Read the model definition and answer for the solid it produces. Units are mm, in the model's axes. A direction names the side the tool comes from. Coordinates: 2 decimals unless noted, no trailing zeros. Write each loop counter-clockwise with the first axis right and the second up, starting at its lowest first coordinate (ties: lowest second). Pieces come first, ordered by that corner, then holes. Notation, with made-up numbers: (79, 78.5) -> (100, 78.5) arc R14 ccw to (100, 85.5) -> close; hole circle Ø4 at (-7, 71). An arc over 180 degrees is marked (long way). Answer as a JSON object with one key per item and string values. Group by question number.
(1) Find section A-A (z = -38.5). Give the vertices of the cut face in (x, y), then the cut area to 3 significant figures.
(2) Find section B-B (x = 160.5). Give the vertices of the cut face in (y, z).
(3) Find section C-C (y = 30.5). Give the vertices of the cut face in (x, z), then the cut area to 3 significant figures.
(4) Which of the six approach directions +Z, -Z, +X, -X, +Y, -Y give full straight-line access (tool end or side, diameter ignored) to faces 5 (the face through (148, 44.45, -50)), 6 (the face through (246.77, 3.13, -29.3)), 7 (the face through (260.63, 27.88, -98.47)), 8 (the face through (254.514, 26.016, -3.131))?
(5) For a pull along Z with two mould halves and no side action, classify faces 1 (the face through (148, 0, -52)), 2 (the face through (246.619, 3.131, -72.715)), 3 (the face through (148, 26, -101.6)), 4 (the face through (148, 25, 0)) as +Z half, -Z half, draft (parallel to the pull), parting line (faces both ways), or undercut.
(6) Straight lines are drawn through the part: L1, parallel to Z at x = 242, y = 2; L2, parallel to Y at x = 287, z = -4; L3, parallel to X at y = 47.25, z = -30.8. For each, find the intervals that lie inside material, in ascending order.
(7) Flat-ended cylindrical pins translate along their axes: P1, Ø9, axis at x = 242, z = -70.8, coming from the -Y side; P2, Ø3.5, axis at x = 255.065, y = 38.835, coming from the +Z side. Find the tip coordinate at first contact, or state that the pin passes through.
Autodesk Inventor part; units mm, degrees
ref_plane "YZ Plane" through (0, 0, 0) normal (1, 0, 0) x (0, 1, 0)
ref_plane "XZ Plane" through (0, 0, 0) normal (0, 1, 0) x (-1, 0, 0)
ref_plane "XY Plane" through (0, 0, 0) normal (0, 0, 1) x (1, 0, 0)
sketch "Sketch1" plane through (0, 0, 0) normal (1, 0, 0) x (0, 1, 0)
  line L0 (0, 0) -> (50.8, 0)
  line L1 (50.8, 0) -> (50.8, -101.6)
  line L2 (50.8, -101.6) -> (0, -101.6)
  line L3 (0, -101.6) -> (0, 0)
  dimension "d0" = 101.6
  dimension "d1" = 50.8
extrude "Extrusion1" add sketch "Sketch1" along normal blind 300
shell "Shell1" thickness 6.35 removed faces 2 at (0, 16.9333, -33.8667) at (300, 16.9333, -33.8667)
sketch "Sketch2" plane through (0, 50.8, 0) normal (0, 1, 0) x (1, 0, 0)
  circle A0 centre (295, 70.8) radius 2
  circle A1 centre (295, 30.8) radius 2
  circle A2 centre (242, 70.8) radius 2
  circle A3 centre (242, 30.8) radius 2
  line L0 (295, 70.8) -> (242, 70.8) construction
  line L1 (242, 70.8) -> (242, 30.8) construction
  line L2 (242, 30.8) -> (295, 30.8) construction
  line L3 (295, 30.8) -> (295, 70.8) construction
  line L4 (300, 101.6) -> (300, 0)
  line L5 (237, 101.6) -> (237, 0)
  line L6 (237, 0) -> (300, 0)
  line L7 (300, 101.6) -> (237, 101.6)
  point P0 (268.5, 0)
  point P1 (268.5, 30.8)
  point P2 (295, 50.8)
  point P3 (300, 50.8)
  dimension "d5" = 4
  dimension "d6" = 63
  dimension "d7" = 40
  dimension "d8" = 53
extrude "Extrusion2" cut sketch "Sketch2" against normal up to surface (6.35 mm away) contours A0 | A1 | A2 | A3
sketch "Sketch3" plane through (0, 0, 0) normal (0, 0, 1) x (1, 0, 0)
  line L0 (297, 44.45) -> (293, 44.45) construction
  line L1 (244, 44.45) -> (240, 44.45) construction
  circle A0 centre (268.5, 25.4) radius 19 construction
  line L2 (300, 50.8) -> (300, 0) construction
  line L3 (293, 44.45) -> (268.5, 25.4) construction
  line L4 (268.5, 25.4) -> (244, 44.45) construction
  circle A1 centre (255.065, 11.965) radius 2
  circle A2 centre (281.935, 11.965) radius 2
  circle A3 centre (281.935, 38.835) radius 2
  circle A4 centre (287.5, 25.4) radius 2
  circle A5 centre (255.065, 38.835) radius 2
  circle A6 centre (249.5, 25.4) radius 2
  line L5 (249.5, 25.4) -> (268.5, 25.4) construction
  line L6 (255.065, 11.965) -> (268.5, 25.4) construction
  circle A7 centre (268.5, 25.4) radius 14
  point P0 (0, 0)
  point P1 (300, 25.4)
  point P2 (300, 25.4)
  dimension "d11" = 38
  dimension "d12" = 4
  dimension "d13" = 45
  dimension "d14" = 28
extrude "Extrusion3" cut sketch "Sketch3" against normal up to surface (6.35 mm away)
sketch "Sketch4" plane through (0, 0, -101.6) normal (0, 0, -1) x (-1, 0, 0)
  circle A0 centre (-268.5, 25.4) radius 14 construction
  circle A1 centre (-268.5, 25.4) radius 8.25
  point P0 (0, 0)
  dimension "d17" = 16.5
extrude "Extrusion4" cut sketch "Sketch4" against normal up to surface (6.35 mm away)
sketch "Sketch5" plane through (0, 0, -101.6) normal (0, -1, 0) x (1, 0, 0)
  circle A0 centre (242, 30.8) radius 2
  circle A1 centre (242, 70.8) radius 2
  circle A2 centre (242, 30.8) radius 5
  circle A3 centre (242, 70.8) radius 5
  point P0 (0, 101.6)
  dimension "d20" = 10
extrude "Extrusion5" cut sketch "Sketch5" against normal up to surface (6.35 mm away) contours A0 | A1 | A2 | A3
properties part number "VERTICALTUBE"
Results below:
{
 "1": {"outline": "(0, 0) -> (300, 0) -> (300, 6.35) -> (0, 6.35) -> close; (0, 44.45) -> (300, 44.45) -> (300, 50.8) -> (0, 50.8) -> close", "area": "3,810 mm2"},
 "2": {"outline": "(0, -101.6) -> (50.8, -101.6) -> (50.8, 0) -> (0, 0) -> close; hole (6.35, -95.25) -> (44.45, -95.25) -> (44.45, -6.35) -> (6.35, -6.35) -> close"},
 "3": {"outline": "(0, -101.6) -> (262.02, -101.6) -> (262.02, -95.25) -> (0, -95.25) -> close; (0, -6.35) -> (255.46, -6.35) -> (255.46, 0) -> (0, 0) -> close; (274.98, -101.6) -> (300, -101.6) -> (300, -95.25) -> (274.98, -95.25) -> close; (281.54, -6.35) -> (300, -6.35) -> (300, 0) -> (281.54, 0) -> close", "area": "3,560 mm2"},
 "4": {"face 5": "+X, -X", "face 6": "-Y", "face 7": "+Z, -Z", "face 8": "+Z"},
 "5": {"face 1": "draft", "face 2": "undercut", "face 3": "-Z half", "face 4": "+Z half"},
 "6": {"L1": "z = -101.6 to -75.8, -65.8 to -35.8, -25.8 to 0", "L2": "y = 0 to 23.46, 27.34 to 50.8", "L3": "x = 0 to 240, 244 to 293, 297 to 300"},
 "7": {"P1": "stops at y = 44.45", "P2": "stops at z = -95.25"}
}
